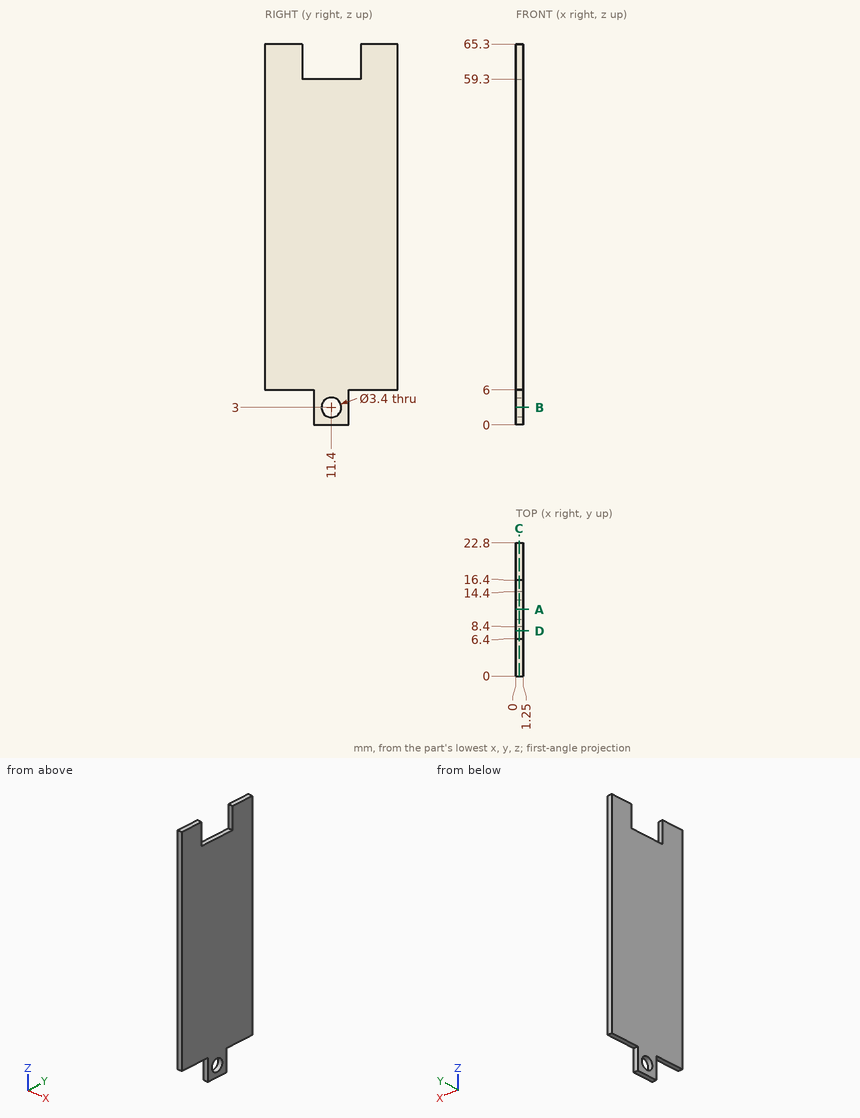
Job drawing, mm, ordinate dimensions from the low corner. One solid piece. Give positions to 0.01 mm unless a question says otherwise; leave off trailing zeros. Loops run counter-clockwise (first coordinate to the right, second up) from the corner with the lowest first, then second, coordinate; pieces in that order, holes last. Notation, with made-up numbers: M 10.25,86 L 48.25,86 A16 cw 48.25,97 Z; hole C -14.5,39 d7. An arc over 180 degrees is marked long. Answer in a Markdown table with one row per item. Add a question column.
Item 1: Band-saw the part on C-C on x = 0.55. Give the cut face in (y, z).
Item 2: Band-saw the part on D-D on y = 7.75. Give the cut face in (x, z), then the cut area to 3 significant figures.
Item 3: Probe probe 1 along Y at (x, z) = (0.8, 3); probe 2 along Y at (x, z) = (0.95, 62.5); probe 3 along Z at (x, y) = (0.6, 3.75). List the from-to ranges inside material, lowest first.
Item 4: Band-saw the part on B-B on z = 3. Give the cut face in (x, y), then the cut area to 3 significant figures.
Item 5: Drop flat-ended pins along their axis: P1, Ø0.6, axis at x = 0.5, y = 11.5, coming from the +Z side; P2, Ø0.6, axis at x = 0.5, z = 4.5, coming from the +Y side; P3, Ø3, axis at y = 11.4, z = 3, coming from the +X side. Give the stop position or say it passes through.
Item 6: Band-saw the part on A-A on y = 11.4. Give the cut face in (x, z).
Reply:
| question | item | result |
|---|---|---|
| 1 | outline | M 0,6 L 8.4,6 L 8.4,0 L 14.4,0 L 14.4,6 L 22.8,6 L 22.8,65.3 L 16.4,65.3 L 16.4,59.3 L 6.4,59.3 L 6.4,65.3 L 0,65.3 Z; hole C 11.4,3 d3.4 |
| 2 | outline | M 0,6 L 1.25,6 L 1.25,59.3 L 0,59.3 Z |
| 2 | area | 66.6 mm^2 |
| 3 | probe 1 | y = 8.4 to 9.7, 13.1 to 14.4 |
| 3 | probe 2 | y = 0 to 6.4, 16.4 to 22.8 |
| 3 | probe 3 | z = 6 to 65.3 |
| 4 | outline | M 0,8.4 L 1.25,8.4 L 1.25,9.7 L 0,9.7 Z; M 0,13.1 L 1.25,13.1 L 1.25,14.4 L 0,14.4 Z |
| 4 | area | 3.25 mm^2 |
| 5 | P1 | stops at z = 59.3 |
| 5 | P2 | stops at y = 14.4 |
| 5 | P3 | passes through |
| 6 | outline | M 0,0 L 1.25,0 L 1.25,1.3 L 0,1.3 Z; M 0,4.7 L 1.25,4.7 L 1.25,59.3 L 0,59.3 Z |
